Source: CAD feature listing. Evaluate the final solid. Frame: model axes, mm. A direction names the side the tool comes from. Give positions to 0.01 mm unless a question says otherwise; leave off trailing zeros. Write each loop counter-clockwise with the first axis right and the second up, starting at its lowest first coordinate (ties: lowest second). Pieces come first, ordered by that corner, then holes. Notation, with made-up numbers: (85.5, 44) - (118.5, 44) arc R20 ccw to (118.5, 79) - close; hole circle Ø6 at (36, 6.25). An arc over 180 degrees is marked (long way). One line per question, with ' | ' between items. Start each with the question number.
(1) Section B-B, the plane x = 0. Return loops of the section in (y, z), plus the area to 3 significant figures.
(2) Section C-C, the plane y = 0.75. Return loops of the section in (x, z), plus the area to 3 significant figures.
(3) Access query for faces 1 (the flat face through (-7, -1, 7.05)), 2 (the flat face through (-7, -1, 12.95)), 3 (the flat face through (-1.2, 2.5, -12.2)). Directions: +Z, -Z, +X, -X, +Y, -Y. A direction counts if a zero-diameter tool reaches every point of the face in a straight line with its end or side. Return the directions, or none.
(4) Section D-D, the plane x = 8.5. Return loops of the section in (y, z).
(5) Ray query, line 1 (Z direction, x = 0, y = 2.4); line 2 (Z direction, x = 0, y = 2.7); line 3 (X direction, y = 1.5, z = 10). Return the intervals inside material, ascending. Write a range as [from, to].
(6) Pin query (flat end, axial travel): pin 1 (0.6 mm diameter, centred on x = -7, y = -1, fed in from -Z); pin 2 (5.5 mm diameter, centred on x = 0, z = 10, fed in from +Y); pin 3 (1.6 mm diameter, centred on x = 6.5, y = -1, fed in from +Z). Return the tip coordinate at first contact, or that it passes through.
(7) Section A-A, the plane z = 10. Return loops of the section in (x, y).
(8) Draft query along X for faces 4 (the flat face through (-10, 1, 0)), 5 (the cylindrical face through (-0.3, 3.01, -12.28)), 6 (the flat face through (0, 4, 0)). Return one class per face: +X half, -X half, draft (parallel to the pull), parting line (faces both ways), or undercut.
```python
from build123d import *

# Parameters (mm, degrees)
ESBO_O1_W                  = 20
ESBO_O1_H                  = 40
RESSALTO_EXTRUS_O1_DEPTH   = 4
ESBO_O2_R                  = 2.3
CORTE_EXTRUS_O1_DEPTH      = 1
CORTE_EXTRUS_O1_DEPTH_BACK = 5
ESBO_O3_W                  = 7
ESBO_O3_H                  = 5.9
RESSALTO_EXTRUS_O2_DEPTH   = 2
CHANFRO1_SIZE              = 0.5
ESBO_O4_R                  = 5
CORTE_EXTRUS_O2_DEPTH      = 2.5


with BuildPart() as part:
    # Esboço1 → Ressalto-extrusão1 (new body)
    with BuildSketch(Plane(origin=(0, 0, 0), x_dir=(1, 0, 0), z_dir=(0, 1, 0))):
        Rectangle(ESBO_O1_W, ESBO_O1_H)
    extrude(amount=RESSALTO_EXTRUS_O1_DEPTH)

    # Esboço2 → Corte-extrusão1 (cut, two sides)
    with BuildSketch(Plane(origin=(0, 4, 0), x_dir=(1, 0, 0), z_dir=(0, 1, 0))) as corte_extrus_o1_sk:
        with Locations((0, 10)):
            Circle(ESBO_O2_R)
        with Locations((0, -10)):
            Circle(ESBO_O2_R)
    extrude(amount=CORTE_EXTRUS_O1_DEPTH, mode=Mode.SUBTRACT)
    extrude(corte_extrus_o1_sk.sketch, amount=-CORTE_EXTRUS_O1_DEPTH_BACK, mode=Mode.SUBTRACT)

    # Esboço3 → Ressalto-extrusão2 (add)
    with BuildSketch(Plane.XZ):
        with Locations((6.5, 10)):
            Rectangle(ESBO_O3_W, ESBO_O3_H)
        with Locations((-6.5, 10)):
            Rectangle(ESBO_O3_W, ESBO_O3_H)
    extrude(amount=RESSALTO_EXTRUS_O2_DEPTH)

    # Chanfro1
    chanfro1_edges = [part.edges().sort_by_distance(p)[0] for p in [
        (-10, 4, 0),
        (0, 4, 20),
        (-2.3, 4, -10),
        (-2.3, 4, 10),
        (10, 4, 0),
        (0, 4, -20),
    ]]
    chamfer(chanfro1_edges, length=CHANFRO1_SIZE)

    # Esboço4 → Corte-extrusão2 (cut)
    with BuildSketch(Plane.XZ):
        with Locations((0, -10)):
            Circle(ESBO_O4_R)
    extrude(amount=-CORTE_EXTRUS_O2_DEPTH, mode=Mode.SUBTRACT)


solid = part.part
```
Check sheet entries:
1) outline: (0, -20) - (3.5, -20) - (4, -19.5) - (4, -12.8) - (3.5, -12.3) - (2.5, -12.3) - (2.5, -15) - (0, -15) - close; (0, -5) - (2.5, -5) - (2.5, -7.7) - (3.5, -7.7) - (4, -7.2) - (4, 7.2) - (3.5, 7.7) - (0, 7.7) - close; (0, 12.3) - (3.5, 12.3) - (4, 12.8) - (4, 19.5) - (3.5, 20) - (0, 20) - close | area: 109 mm²
2) outline: (-10, -20) - (10, -20) - (10, 20) - (-10, 20) - close; hole circle Ø10 at (0, -10); hole circle Ø4.6 at (0, 10) | area: 705 mm²
3) face 1: -Z, +X, -X, -Y | face 2: +Z, +X, -X, -Y | face 3: -Y
4) outline: (-2, 7.05) - (0, 7.05) - (0, -20) - (3.5, -20) - (4, -19.5) - (4, 19.5) - (3.5, 20) - (0, 20) - (0, 12.95) - (-2, 12.95) - close
5) line 1: [-20, -15], [-5, 7.7], [12.3, 20] | line 2: [-20, -12.3], [-7.7, 7.7], [12.3, 20] | line 3: [-10, -2.3], [2.3, 10]
6) pin 1: z = 7.05 | pin 2: y = 3.95 | pin 3: z = 12.95
7) outline: (-10, -2) - (-3, -2) - (-3, 0) - (-2.3, 0) - (-2.3, 3.5) - (-2.8, 4) - (-9.5, 4) - (-10, 3.5) - close; (2.3, 0) - (3, 0) - (3, -2) - (10, -2) - (10, 3.5) - (9.5, 4) - (2.8, 4) - (2.3, 3.5) - close
8) face 4: -X half | face 5: undercut | face 6: draft
